Autodesk Inventor part; units mm, degrees
ref_plane "YZ Plane" through (0, 0, 0) normal (1, 0, 0) x (0, 1, 0)
ref_plane "XZ Plane" through (0, 0, 0) normal (0, 1, 0) x (-1, 0, 0)
ref_plane "XY Plane" through (0, 0, 0) normal (0, 0, 1) x (1, 0, 0)
sketch "Sketch1" plane through (0, 0, 0) normal (0, 1, 0) x (-1, 0, 0)
  line L0 (-25, -34) -> (25, -34)
  line L1 (25, -34) -> (25, 34)
  line L2 (25, 34) -> (-25, 34)
  line L3 (-25, 34) -> (-25, -34)
  line L4 (-25, -34) -> (25, 34) construction
  line L5 (25, -34) -> (-25, 34) construction
  point P0 (0, 0)
  dimension "d0" = 50
  dimension "d1" = 68
extrude "Extrusion1" add sketch "Sketch1" along normal blind 4.5
sketch "Sketch2" plane through (0, 4.5, 0) normal (0, 1, 0) x (1, 0, 0)
  circle A0 centre (-15, 15) radius 1
  circle A1 centre (15, 15) radius 1
  circle A2 centre (15, -15) radius 1
  circle A3 centre (-15, -15) radius 1
  point P0 (0, 0)
  dimension "d4" = 2
  dimension "d5" = 2
  dimension "d6" = 2
  dimension "d7" = 2
extrude "Extrusion2" cut sketch "Sketch2" against normal blind 4.5
sketch "Sketch3" plane through (0, 0, 0) normal (0, -1, 0) x (1, 0, 0)
  circle A0 centre (15, 15) radius 2.5
  circle A1 centre (-15, 15) radius 2.5
  circle A2 centre (-15, -15) radius 2.5
  circle A3 centre (15, -15) radius 2.5
  circle A4 centre (15, -15) radius 1
  circle A5 centre (15, 15) radius 1
  circle A6 centre (15, 15) radius 1
  circle A7 centre (-15, 15) radius 1
  circle A8 centre (-15, 15) radius 1
  circle A9 centre (-15, -15) radius 1
  point P0 (0, 0)
  dimension "d10" = 5
  dimension "d11" = 5
  dimension "d12" = 5
extrude "Extrusion3" add sketch "Sketch3" along normal blind 5
fillet "Fillet1" radius 2 4 edges at (-25, 2.25, 34) (25, 2.25, 34) (25, 2.25, -34) (-25, 2.25, -34)
fillet "Fillet2" radius 1 4 edges at (12.5, 0, -15) (12.5, 0, 15) (-17.5, 0, -15) (-17.5, 0, 15)
properties part number "feste"
For this review, take the finished solid that the model builds, in its own axes (mm). A direction names the side the tool comes from. Give positions to 0.01 mm unless a question says otherwise; leave off trailing zeros. Loops run counter-clockwise (first coordinate to the right, second up) from the corner with the lowest first, then second, coordinate; pieces in that order, holes last. Notation, with made-up numbers: (-0.5, 60.25) - (57.5, 60.25) arc R20 cw to (57.5, 76.25) - close; hole circle Ø3 at (-19, -3). An arc over 180 degrees is marked (long way). Write each question's results on one line, items separated by ' | '.
(1) Take a section at A-A (z = -15). Give the boundary of the cut face in (x, y).
Conclusion:
outline: (-25, 0) - (-18.5, 0) arc R1 cw to (-17.5, -1) - (-17.5, -5) - (-16, -5) - (-16, 4.5) - (-25, 4.5) - close; (-14, -5) - (-12.5, -5) - (-12.5, -1) arc R1 cw to (-11.5, 0) - (11.5, 0) arc R1 cw to (12.5, -1) - (12.5, -5) - (14, -5) - (14, 4.5) - (-14, 4.5) - close; (16, -5) - (17.5, -5) - (17.5, -1) arc R1 cw to (18.5, 0) - (25, 0) - (25, 4.5) - (16, 4.5) - close
(2) Draft analysis for pull direction Z (two halves, no side actions). For faces 1 (the cylindrical face through (24.43, 2.28, -33.4)), 2 (the flat face through (0, 2, 34)), 3 (the flat face through (25, 2, 0)), 4 (the cylindrical face through (-17, -3, -13.5)), state which applies: +Z half, -Z half, draft (parallel to the pull), parting line (faces both ways), or undercut.
Conclusion:
face 1: -Z half | face 2: +Z half | face 3: draft | face 4: undercut
(3) For faces 5 (the flat face through (0, 0, 0)), 6 (the flat face through (-25, 2, 0)), list the 3-axis set-ups (+Z, -Z, +X, -X, +Y, -Y) from which the entire face can be reached by the end or side of a thin tool; tool diameter is ignored.
Conclusion:
face 5: -Y | face 6: +Z, -Z, -X, +Y, -Y
(4) For line 1 along X through (y, z) = (1.75, 15); line 2 along Z through (x, y) = (15, -2.25); line 3 along Z through (x, y) = (15, 0.5), list the stretches that pass through material, from the lowest coordinate up.
Conclusion:
line 1: -25 to -16, -14 to 14, 16 to 25 | line 2: -17.5 to -16, -14 to -12.5, 12.5 to 14, 16 to 17.5 | line 3: -34 to -16, -14 to 14, 16 to 34
(5) Take a section at B-B (x = -15). Give the boundary of the cut face in (y, z).
Conclusion:
outline: (-5, -17.5) - (-1, -17.5) arc R1 cw to (0, -18.5) - (0, -34) - (4.5, -34) - (4.5, -16) - (-5, -16) - close; (-5, -14) - (4.5, -14) - (4.5, 14) - (-5, 14) - (-5, 12.5) - (-1, 12.5) arc R1 cw to (0, 11.5) - (0, -11.5) arc R1 cw to (-1, -12.5) - (-5, -12.5) - close; (-5, 16) - (4.5, 16) - (4.5, 34) - (0, 34) - (0, 18.5) arc R1 cw to (-1, 17.5) - (-5, 17.5) - close
(6) For pin 1 Ø1.5 at (x, z) = (-0.5, -5.5) entering from -Y; pin 2 Ø2 at (x, y) = (14.5, -3) entering from -Z, all flat-tipped, find the tip position at first contact; note any pin that passes through.
Conclusion:
pin 1: y = 0 | pin 2: z = -17.5
